from build123d import *

# Parameters (mm, degrees)
F0_W     = 450
F0_H     = 375
F0_W_2   = 25
F0_H_2   = 25
F1_DEPTH = 25
F3_W     = 25
F3_H     = 35
F4_DEPTH = 25
F5_R     = 5


with BuildPart() as f1:
    # F0 (on Top) → F1 (new body)
    with BuildSketch(Plane.XY):
        with Locations((-225, 46.5578983041)):
            Rectangle(F0_W, F0_H)
        with Locations((-387.5, -103.4421016959)):
            Rectangle(F0_W_2, F0_H_2, mode=Mode.SUBTRACT)
        with Locations((-387.5, -53.4421016959)):
            Rectangle(F0_W_2, F0_H_2, mode=Mode.SUBTRACT)
        with Locations((-387.5, -3.4421016959)):
            Rectangle(F0_W_2, F0_H_2, mode=Mode.SUBTRACT)
        with Locations((-387.5, 46.5578983041)):
            Rectangle(F0_W_2, F0_H_2, mode=Mode.SUBTRACT)
        with Locations((-387.5, 96.5578983041)):
            Rectangle(F0_W_2, F0_H_2, mode=Mode.SUBTRACT)
        with Locations((-387.5, 146.5578983041)):
            Rectangle(F0_W_2, F0_H_2, mode=Mode.SUBTRACT)
        with Locations((-387.5, 196.5578983041)):
            Rectangle(F0_W_2, F0_H_2, mode=Mode.SUBTRACT)
    extrude(amount=F1_DEPTH)

    # F2: F1 across face


with BuildPart() as f1_1:
    add(f1.part)
    add(f1.part.mirror(Plane(origin=(0, 46.5578983041, 12.5), x_dir=(0, 1, 0), z_dir=(1, 0, 0))))

    # F3 (on face) → F4 (cut)
    with BuildSketch(Plane(origin=(0, 0, 0), x_dir=(1, 0, 0), z_dir=(0, 0, -1))):
        with Locations((0, -166.5578983041)):
            Rectangle(F3_W, F3_H)
        with Locations((0, 73.4421016959)):
            Rectangle(F3_W, F3_H)
    extrude(amount=-F4_DEPTH, mode=Mode.SUBTRACT)

    # F5
    f5_edges = [f1_1.edges().sort_by_distance(p)[0] for p in [
        (0, 234.057898, 25),
        (450, 46.557898, 25),
        (-450, 46.557898, 25),
    ]]
    fillet(f5_edges, radius=F5_R)


solid = f1_1.part
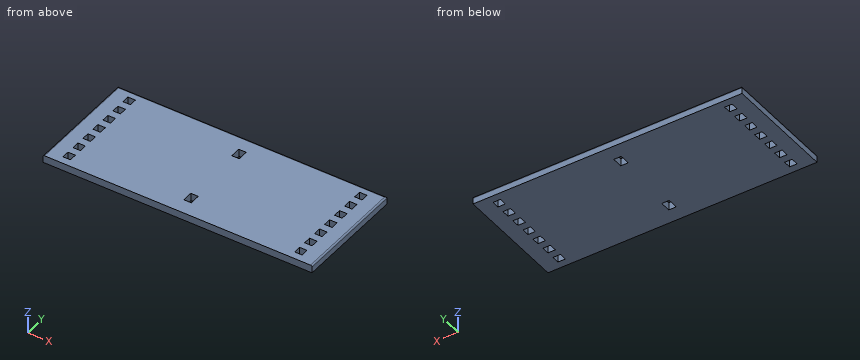
Can you work these out from the model? Positions are in its coordinate system, mm. Coordinates: 2 decimals unless noted, no trailing zeros. Order: outer loops, then holes, each group sorted by start corner. A loop starts at its lowest first (then second) coordinate and runs counter-clockwise, first axis right, second up. Notation, with made-up numbers: (74, 86.5) - (124, 86.5) arc R26 cw to (124, 105.5) - close; hole circle Ø3 at (8.5, -5). An arc over 180 degrees is marked (long way). Answer as a JSON object with one key per item and string values. Group by question number.
Q1. Imagine slicing it at C-C (z = 15). Give the number of separate pieces and of enclosed holes in the cut face, and give its area (3 significant figures).
Q2. Imagine slicing it at B-B (y = -100.5). Please give me the cut outline in (x, z), and give its area (3 significant figures).
Q3. I need wall thicknesses on line 1 (Y direction, x = 0, z = 1); line 2 (X direction, y = 88, z = 6); line 3 (X direction, y = 196, z = 21.25). Which ranges of each line are inside material? Lowest first, please. Write a range as from..to.
Q4. Imagine slicing it at A-A (y = 168). Please give me the cut outline in (x, z), and give its area (3 significant figures).
Determined:
{
 "1": {"separate pieces": "1", "enclosed holes": "16", "area": "327,000 mm2"},
 "2": {"outline": "(-450, 0) - (-400, 0) - (-400, 25) - (-445, 25) arc R5 ccw to (-450, 20) - close; (-375, 0) - (375, 0) - (375, 25) - (-375, 25) - close; (400, 0) - (450, 0) - (450, 20) arc R5 ccw to (445, 25) - (400, 25) - close", "area": "21,200 mm2"},
 "3": {"line 1": "y = -140.94..-90.94, -55.94..149.06, 184.06..234.06", "line 2": "x = -450..-400, -375..375, 400..450", "line 3": "x = -449.84..-400, -375..375, 400..449.84"},
 "4": {"outline": "(-450, 0) - (-12.5, 0) - (-12.5, 25) - (-445, 25) arc R5 ccw to (-450, 20) - close; (12.5, 0) - (450, 0) - (450, 20) arc R5 ccw to (445, 25) - (12.5, 25) - close", "area": "21,900 mm2"}
}
